Build history of the part. All positions in model axes, mm. A direction names the side the tool comes from. Give positions to 0.01 mm unless a question says otherwise; leave off trailing zeros. Order: outer loops, then holes, each group sorted by start corner. A loop starts at its lowest first (then second) coordinate and runs counter-clockwise, first axis right, second up. Notation, with made-up numbers: M 5,48 L 62,48 A30 ccw 62,83 Z; hole C -26.5,-30 d6. An arc over 180 degrees is marked long. One line per item, written item: value. Start each with the question number.
from build123d import *

# Parameters (mm, degrees)
CROQUIS2_W              = 83
CROQUIS2_H              = 100
CROQUIS2_W_2            = 76
CROQUIS2_H_2            = 93.334161502
SALIENTE_EXTRUIR1_DEPTH = 43
CROQUIS3_W              = 83
CROQUIS3_H              = 3
SALIENTE_EXTRUIR2_DEPTH = 100
CROQUIS4_W              = 69
CROQUIS4_H              = 16
CORTAR_EXTRUIR3_DEPTH   = 10
SALIENTE_EXTRUIR3_DEPTH = 3
CROQUIS6_R              = 1.5
CORTAR_EXTRUIR4_DEPTH   = 13
REDONDEO1_R             = 3
REDONDEO2_R             = 1


with BuildPart() as part:
    # Croquis2 → Saliente-Extruir1 (new body)
    with BuildSketch(Plane(origin=(0, -3.101295798, 0), x_dir=(1, 0, 0), z_dir=(0, 1, 0))):
        with Locations((-13.660303869, -172.250641144)):
            Rectangle(CROQUIS2_W, CROQUIS2_H)
        with Locations((-13.160303869, -171.917721895)):
            Rectangle(CROQUIS2_W_2, CROQUIS2_H_2, mode=Mode.SUBTRACT)
    extrude(amount=SALIENTE_EXTRUIR1_DEPTH)

    # Croquis3 → Saliente-Extruir2 (add)
    with BuildSketch(Plane.XY.offset(222.250641144)):
        with Locations((-13.660303869, 41.398704202)):
            Rectangle(CROQUIS3_W, CROQUIS3_H)
    extrude(amount=-SALIENTE_EXTRUIR2_DEPTH)

    # Croquis4 → Cortar-Extruir3 (cut)
    with BuildSketch(Plane.XY.offset(222.250641144)):
        with Locations((-13.660303869, 4.898704202)):
            Rectangle(CROQUIS4_W, CROQUIS4_H)
    extrude(amount=-CORTAR_EXTRUIR3_DEPTH, mode=Mode.SUBTRACT)

    # Croquis5 → Saliente-Extruir3 (add)
    with BuildSketch(Plane(origin=(0, -3.101295798, 0), x_dir=(1, 0, 0), z_dir=(0, 1, 0))):
        with BuildLine():
            Line((-58.160303869, -169.250641144), (-55.160303869, -169.250641144))
            Line((-55.160303869, -169.250641144), (-55.160303869, -175.250641144))
            Line((-55.160303869, -175.250641144), (-58.160303869, -175.250641144))
            ThreePointArc((-58.160303869, -175.250641144), (-61.160303869, -172.250641144), (-58.160303869, -169.250641144))
        make_face()
        with BuildLine():
            Line((-16.660303869, -119.250641144), (-16.660303869, -122.250641144))
            Line((-16.660303869, -122.250641144), (-10.660303869, -122.250641144))
            Line((-10.660303869, -122.250641144), (-10.660303869, -119.250641144))
            ThreePointArc((-10.660303869, -119.250641144), (-13.660303869, -116.250641144), (-16.660303869, -119.250641144))
        make_face()
        with BuildLine():
            Line((30.839696131, -169.250641144), (27.839696131, -169.250641144))
            Line((27.839696131, -169.250641144), (27.839696131, -175.250641144))
            Line((27.839696131, -175.250641144), (30.839696131, -175.250641144))
            ThreePointArc((30.839696131, -175.250641144), (33.839696131, -172.250641144), (30.839696131, -169.250641144))
        make_face()
    extrude(amount=SALIENTE_EXTRUIR3_DEPTH)

    # Croquis6 → Cortar-Extruir4 (cut)
    with BuildSketch(Plane(origin=(0, -0.101295798, 0), x_dir=(1, 0, 0), z_dir=(0, 1, 0))):
        with Locations((30.839696131, -172.250641144)):
            Circle(CROQUIS6_R)
        with Locations((-13.660303869, -119.250641144)):
            Circle(CROQUIS6_R)
        with Locations((-58.160303869, -172.250641144)):
            Circle(CROQUIS6_R)
    extrude(amount=-CORTAR_EXTRUIR4_DEPTH, mode=Mode.SUBTRACT)

    # Redondeo1
    redondeo1_edges = [part.edges().sort_by_distance(p)[0] for p in [
        (-13.660303869, 42.898704202, 122.250641144),
        (-55.160303869, 42.898704202, 172.250641144),
        (27.839696131, 42.898704202, 172.250641144),
        (-13.660303869, 42.898704202, 222.250641144),
        (-55.160303869, 19.898704202, 122.250641144),
        (27.839696131, 19.898704202, 122.250641144),
        (27.839696131, 19.898704202, 222.250641144),
        (-55.160303869, 19.898704202, 222.250641144),
    ]]
    fillet(redondeo1_edges, radius=REDONDEO1_R)

    # Redondeo2
    redondeo2_edges = [part.edges().sort_by_distance(p)[0] for p in [
        (24.839696131, 18.398704202, 218.584802646),
        (24.839696131, 18.398704202, 125.250641144),
        (-51.160303869, 18.398704202, 125.250641144),
        (-51.160303869, 18.398704202, 218.584802646),
        (24.839696131, 39.898704202, 171.917721895),
        (-13.160303869, 39.898704202, 125.250641144),
        (-51.160303869, 39.898704202, 171.917721895),
        (-13.160303869, 39.898704202, 218.584802646),
    ]]
    fillet(redondeo2_edges, radius=REDONDEO2_R)


solid = part.part
1) Slice it at C-C (x = -8.5). List the corners of the cut face in (y, z).
2) Slice it at A-A (y = 27.5). List the corners of the cut face in (x, z).
3) Pull direction X, two halves, no side cores. Call faces 6 (the flat face through (-53, -3.101, 173)), 7 (the flat face through (20.84, 5, 220)), 8 (the cylindrical face through (-13.59, -1.62, 116.25)): pulls with the +X half, pulls with the -X half, needs draft (parallel to the pull), parting line crosses it, or undercut.
4) Drill centre lines: line 1 (Z direction, x = 21.5, y = 25.5); line 2 (X direction, y = 0.5, z = 137); line 3 (Y direction, x = 22.5, z = 183.5). Where is each one in solid material? Low to high.
5) Slice it at B-B (z = 211.5). List the corners of the cut face in (x, y), plus the area to 3 significant figures.
6) Tool access for faces 1 (the flat face through (-57, -2, 175.251)), 2 (the flat face through (-14, 18, 125.251)), 3 (the flat face through (-57, -0.101, 171)), 4 (the flat face through (-14, 12.899, 220)), 5 (the flat face through (-14, -0.101, 121)): list every direction of +Z, -Z, +X, -X, +Y, -Y with a clear straight run to the whole face (end or side of a thin tool).
7) Drop flat-ended pins along their axis: P1, Ø2.5, axis at x = -57.5, y = -2, coming from the +Z side; P2, Ø22, axis at x = -15.5, z = 172, coming from the -Y side; P3, Ø1.8, axis at x = -57.5, z = 173, coming from the +Y side; P4, Ø1.8, axis at x = 30.84, z = 172.25, coming from the -Y side. Give the stop position or say it passes through.
Results list:
1. outline: M -3.1,122.25 L 39.9,122.25 A3 ccw 42.9,125.25 L 42.9,219.25 A3 ccw 39.9,222.25 L 12.9,222.25 L 12.9,218.58 L 38.9,218.58 A1 cw 39.9,217.58 L 39.9,126.25 A1 cw 38.9,125.25 L -3.1,125.25 Z
2. outline: M -55.16,125.25 A3 ccw -52.16,122.25 L 24.84,122.25 A3 ccw 27.84,125.25 L 27.84,219.25 A3 ccw 24.84,222.25 L -52.16,222.25 A3 ccw -55.16,219.25 Z; hole M -51.16,126.25 A1 ccw -50.16,125.25 L 23.84,125.25 A1 ccw 24.84,126.25 L 24.84,217.58 A1 ccw 23.84,218.58 L -50.16,218.58 A1 ccw -51.16,217.58 Z
3. face 6: needs draft
3. face 7: undercut
3. face 8: parting line crosses it
4. line 1: z = 122.25 to 125.25, 218.58 to 222.25
4. line 2: x = -55.16 to -51.16, 24.84 to 27.84
4. line 3: y = 39.9 to 42.9
5. outline: M -55.16,-3.1 L -51.16,-3.1 L -51.16,38.9 A1 cw -50.16,39.9 L 23.84,39.9 A1 cw 24.84,38.9 L 24.84,-3.1 L 27.84,-3.1 L 27.84,39.9 A3 ccw 24.84,42.9 L -52.16,42.9 A3 ccw -55.16,39.9 Z
5. area: 547 mm²
6. face 1: +Z, -X, +Y, -Y
6. face 2: -Y
6. face 3: +Z, -Z, -X, +Y
6. face 4: +Z, -Y
6. face 5: -Z, +X, -X, +Y
7. P1: stops at z = 175.25
7. P2: stops at y = 39.9
7. P3: stops at y = -0.1
7. P4: passes through
